Check sheet for the modelled part. Datum: model origin and axes. Units: mm. A direction names the side the tool comes from. Give positions to 0.01 mm unless a question says otherwise; leave off trailing zeros. Order: outer loops, then holes, each group sorted by start corner. A loop starts at its lowest first (then second) coordinate and runs counter-clockwise, first axis right, second up. Notation, with made-up numbers: (-14.5, 13.25) - (-10.5, 13.25) arc R13 cw to (-10.5, 34.25) - close; hole circle Ø1 at (17.5, 23). An arc over 180 degrees is marked (long way). Answer in a Markdown table with one row per item.
from build123d import *

# Parameters (mm, degrees)
SKETCH2_W           = 36
SKETCH2_H           = 42
BOSS_EXTRUDE1_DEPTH = 8
CUT_EXTRUDE1_DEPTH  = 10
CUT_EXTRUDE2_DEPTH  = 10
SKETCH5_W           = 25.353942038
SKETCH5_H           = 1.695405108
CUT_EXTRUDE3_DEPTH  = 25
SKETCH6_R           = 4.125
CUT_EXTRUDE4_DEPTH  = 7.1
SKETCH7_W           = 0.63
SKETCH7_H           = 8
SKETCH7_W_2         = 0.620319398
BOSS_EXTRUDE2_DEPTH = 42


with BuildPart() as part:
    # Sketch2 → Boss-Extrude1 (new body)
    with BuildSketch(Plane.XY):
        with Locations((-1.487179487, 11.461538462)):
            Rectangle(SKETCH2_W, SKETCH2_H)
    extrude(amount=BOSS_EXTRUDE1_DEPTH)

    # Sketch3 → Cut-Extrude1 (cut)
    with BuildSketch(Plane(origin=(0, 32.461538462, 0), x_dir=(1, 0, 0), z_dir=(0, 1, 0))):
        Polygon((-18.212179487, 0), (-18.882052468, -2.5), (-15.042306506, -2.5), (-15.712179487, 0), align=None)
        Polygon((-18.212179487, -8), (-18.882052468, -5.5), (-15.042306506, -5.5), (-15.712179487, -8), align=None)
        Polygon((15.237820513, 0), (15.907693494, -2.5), (12.067947532, -2.5), (12.737820513, 0), align=None)
        Polygon((15.237820513, -8), (15.907693494, -5.5), (12.067947532, -5.5), (12.737820513, -8), align=None)
    extrude(amount=-CUT_EXTRUDE1_DEPTH, mode=Mode.SUBTRACT)

    # Sketch4 → Cut-Extrude2 (cut)
    with BuildSketch(Plane.XY.offset(8)):
        with BuildLine():
            Line((-10.823469947, 32.461538462), (7.849110972, 32.461538462))
            Line((7.849110972, 32.461538462), (7.849110972, 21.461538462))
            ThreePointArc((7.849110972, 21.461538462), (-1.487179487, 12.125248002), (-10.823469947, 21.461538462))
            Line((-10.823469947, 21.461538462), (-10.823469947, 32.461538462))
        make_face()
    extrude(amount=-CUT_EXTRUDE2_DEPTH, mode=Mode.SUBTRACT)

    # Sketch5 → Cut-Extrude3 (cut)
    with BuildSketch(Plane(origin=(0, 32.461538462, 0), x_dir=(1, 0, 0), z_dir=(0, 1, 0))):
        with Locations((-1.487179487, -4)):
            Rectangle(SKETCH5_W, SKETCH5_H)
    extrude(amount=-CUT_EXTRUDE3_DEPTH, mode=Mode.SUBTRACT)

    # Sketch6 → Cut-Extrude4 (cut)
    with BuildSketch(Plane.XY.offset(8)):
        with Locations((-1.491860089, 6.461538462)):
            Circle(SKETCH6_R)
    extrude(amount=-CUT_EXTRUDE4_DEPTH, mode=Mode.SUBTRACT)

    # Sketch7 → Boss-Extrude2 (add)
    with BuildSketch(Plane(origin=(0, 32.461538462, 0), x_dir=(1, 0, 0), z_dir=(0, 1, 0))):
        with Locations((-19.802179487, -4)):
            Rectangle(SKETCH7_W, SKETCH7_H)
        with Locations((16.822980212, -4)):
            Rectangle(SKETCH7_W_2, SKETCH7_H)
    extrude(amount=-BOSS_EXTRUDE2_DEPTH)


solid = part.part
(1) Cross-section at B-B, the plane z = 2. Record the cut outline in (x, y) (3 decimals).
Geometry says:
| item | result |
|---|---|
| outline | (-20.117, -9.538) - (17.133, -9.538) - (17.133, 32.462) - (15.774, 32.462) - (15.774, 22.462) - (12.202, 22.462) - (12.202, 32.462) - (7.849, 32.462) - (7.849, 21.462) arc R9.336 cw to (-10.823, 21.462) - (-10.823, 32.462) - (-15.176, 32.462) - (-15.176, 22.462) - (-18.748, 22.462) - (-18.748, 32.462) - (-20.117, 32.462) - close; hole circle Ø8.25 at (-1.492, 6.462) |
(2) Cross-section at D-D, the plane z = 4.25. Record the cut outline in (x, y) (3 decimals), then the cut area to 3 significant figures.
Geometry says:
| item | result |
|---|---|
| outline | (-20.117, -9.538) - (17.133, -9.538) - (17.133, 32.462) - (11.19, 32.462) - (11.19, 7.462) - (2.51, 7.462) arc R4.125 cw (long way) to (-5.494, 7.462) - (-14.164, 7.462) - (-14.164, 32.462) - (-20.117, 32.462) - close |
| area | 896 mm² |
(3) Cross-section at C-C, the plane x = -0.5. Record the cut outline in (y, z).
Geometry says:
| item | result |
|---|---|
| outline | (-9.54, 0) - (12.18, 0) - (12.18, 3.15) - (10.47, 3.15) - (10.47, 0.9) - (2.46, 0.9) - (2.46, 8) - (-9.54, 8) - close; (10.47, 4.85) - (12.18, 4.85) - (12.18, 8) - (10.47, 8) - close |
(4) Access from +Z, -Z, +X, -X, +Y, -Y to the whole of each face (thin tool, end or side, straight path). Record for faces 1 (the flat face through (7.849, 27, 6)), 2 (the flat face through (-2, 7, 0)), 3 (the flat face through (-18.54, 27.53, 1.23)).
Geometry says:
| item | result |
|---|---|
| face 1 | +Z, -Z, +Y |
| face 2 | -Z, +X, -X, +Y, -Y |
| face 3 | +Y |
(5) Mould release check, pull along X, two halves, no side actions. Record for faces 4 (the flat face through (-2, -9.538, 4)), 5 (the cylindrical face through (-1.282, 12.128, 6.446)): pulls with the +X half, pulls with the -X half, needs draft (parallel to the pull), parting line crosses it, or undercut.
Geometry says:
| item | result |
|---|---|
| face 4 | needs draft |
| face 5 | undercut |
(6) Thickness scan on L1, parallel to Z at x = 8.5, y = 19.5; L2, parallel to X at y = 15.5, z = 3.5; L3, parallel to X at y = 31.5, z = 0.75. Record the ranges inside material, lowest first.
Geometry says:
| item | result |
|---|---|
| L1 | 0 to 3.15, 4.85 to 8 |
| L2 | -20.12 to -14.16, 11.19 to 17.13 |
| L3 | -20.12 to -18.41, -15.51 to -10.82, 7.85 to 12.54, 15.44 to 17.13 |
(7) Gauge pin test, flat ends, axial feed: P1, Ø1.4, axis at x = 6, z = 4, coming from the +Y side; P2, Ø9, axis at x = -2.5, y = 7.5, coming from the +Z side; P3, Ø1.2, axis at x = -16.5, z = 7, coming from the +Y side; P4, Ø3, axis at x = -5.5, z = 2, coming from the +Y side. Record the tip position at first contact, or that the pin passes through.
Geometry says:
| item | result |
|---|---|
| P1 | y = 7.46 |
| P2 | z = 8 |
| P3 | y = 22.46 |
| P4 | y = 13.93 |
